from build123d import *
from OCP.BRepFilletAPI import BRepFilletAPI_MakeFillet
from build123d.topology import SkipClean

# Parameters (mm, degrees)
SKETCH2_R               = 43
SKETCH2_R_2             = 40
BOSS_EXTRUDE1_DEPTH     = 48
SKETCH3_R               = 40
BOSS_EXTRUDE2_DEPTH     = 8.5
CUT_EXTRUDE1_DEPTH      = 71.924255371
CUT_EXTRUDE1_DEPTH_BACK = 71.924255371
SKETCH4_W               = 41
SKETCH4_H               = 21
CUT_EXTRUDE2_DEPTH      = 5
BOSS_EXTRUDE3_START     = 3
SKETCH6_W               = 120
SKETCH6_H               = 110
SKETCH6_R               = 40
BOSS_EXTRUDE3_DEPTH     = 3
FILLET1_R               = 3
FILLET1_R_2             = 1
SKETCH7_R               = 2.1
SKETCH7_W               = 8
SKETCH7_H               = 4
CUT_EXTRUDE3_DEPTH      = 3


with BuildPart() as part:
    # Sketch2 → Boss-Extrude1 (new body)
    with BuildSketch(Plane(origin=(0, 0, 0), x_dir=(1, 0, 0), z_dir=(0, 1, 0))):
        with Locations(Location((0, 0, 0), (0, 0, 270))):
            Circle(SKETCH2_R)
        with Locations(Location((0, 0, 0), (0, 0, 270))):
            Circle(SKETCH2_R_2, mode=Mode.SUBTRACT)
    extrude(amount=BOSS_EXTRUDE1_DEPTH)

    # Sketch3 → Boss-Extrude2 (add)
    with BuildSketch(Plane(origin=(0, 28, 0), x_dir=(1, 0, 0), z_dir=(0, 1, 0))):
        with Locations(Location((0, 0, 0), (0, 0, 270))):
            Circle(SKETCH3_R)
    extrude(amount=BOSS_EXTRUDE2_DEPTH)

    # Sketch4 → Cut-Extrude1 (cut, two sides: drawn at the far end of the back side and taken through both)
    with BuildSketch(Plane(origin=(0, 36.5, 0), x_dir=(1, 0, 0), z_dir=(0, 1, 0)).offset(-CUT_EXTRUDE1_DEPTH_BACK)):
        with BuildLine():
            Line((14, 6.75), (16, 6.75))
            ThreePointArc((16, 6.75), (17.75, 5), (16, 3.25))
            Line((16, 3.25), (14, 3.25))
            ThreePointArc((14, 3.25), (12.25, 5), (14, 6.75))
        make_face()
        with Locations((-10, 0)):
            Rectangle(SKETCH4_W, SKETCH4_H)
        with BuildLine():
            Line((-36, 6.75), (-34, 6.75))
            ThreePointArc((-34, 6.75), (-32.25, 5), (-34, 3.25))
            Line((-34, 3.25), (-36, 3.25))
            ThreePointArc((-36, 3.25), (-37.75, 5), (-36, 6.75))
        make_face()
        with BuildLine():
            Line((-36, -3.25), (-34, -3.25))
            ThreePointArc((-34, -3.25), (-32.25, -5), (-34, -6.75))
            Line((-34, -6.75), (-36, -6.75))
            ThreePointArc((-36, -6.75), (-37.75, -5), (-36, -3.25))
        make_face()
        with BuildLine():
            Line((14, -6.75), (16, -6.75))
            ThreePointArc((16, -6.75), (17.75, -5), (16, -3.25))
            Line((16, -3.25), (14, -3.25))
            ThreePointArc((14, -3.25), (12.25, -5), (14, -6.75))
        make_face()
    extrude(amount=CUT_EXTRUDE1_DEPTH + CUT_EXTRUDE1_DEPTH_BACK, mode=Mode.SUBTRACT)

    # Sketch5 → Cut-Extrude2 (cut)
    with BuildSketch(Plane(origin=(43, 0, 0), x_dir=(0, 0, -1), z_dir=(1, 0, 0))):
        with BuildLine():
            Line((-6, 17), (6, 17))
            ThreePointArc((6, 17), (8, 15), (6, 13))
            Line((6, 13), (-6, 13))
            ThreePointArc((-6, 13), (-8, 15), (-6, 17))
        make_face()
    extrude(amount=-CUT_EXTRUDE2_DEPTH, mode=Mode.SUBTRACT)

    # Sketch6 → Boss-Extrude3 (add)
    with SkipClean():  # the faces are left unmerged after this step: merging them gives an invalid solid
        with BuildSketch(Plane.XZ.offset(BOSS_EXTRUDE3_START)):
            Rectangle(SKETCH6_W, SKETCH6_H)
            with Locations(Location((0, 0, 0), (0, 0, 270))):
                Circle(SKETCH6_R, mode=Mode.SUBTRACT)
        extrude(amount=-BOSS_EXTRUDE3_DEPTH)

    # Fillet1
    fillet1_edges_1 = [part.edges().sort_by_distance(p)[0] for p in [
        (0, 48, -43),
        (0, 0, -43),
    ]]
    fillet1_edges_2 = [part.edges().sort_by_distance(p)[0] for p in [
        (0, 0, 55),
        (60, 0, 0),
        (-60, 0, 0),
        (0, 0, -55),
    ]]
    fillet1 = BRepFilletAPI_MakeFillet(part.part.solid().wrapped)
    for e in fillet1_edges_1:
        fillet1.Add(FILLET1_R - 0.0001, e.wrapped)
    for e in fillet1_edges_2:
        fillet1.Add(FILLET1_R_2 - 0.0001, e.wrapped)
    add(Compound.cast(fillet1.Shape()), mode=Mode.REPLACE)  # a hair under: the kernel refuses the full size

    # Sketch7 → Cut-Extrude3 (cut)
    with BuildSketch(Plane(origin=(0, 0, 0), x_dir=(1, 0, 0), z_dir=(0, 1, 0))):
        with Locations(Location((-41.5, 43, 0), (0, 0, 270))):
            Circle(SKETCH7_R)
        with Locations(Location((43.5, 22.5, 0), (0, 0, 270))):
            Circle(SKETCH7_R)
        with Locations(Location((43.5, -22.5, 0), (0, 0, 270))):
            Circle(SKETCH7_R)
        with Locations(Location((-41.5, -43, 0), (0, 0, 270))):
            Circle(SKETCH7_R)
        with Locations(Location((48.1, 0, 0), (0, 0, 270))):
            Circle(SKETCH7_R)
        with Locations((-49, 25.6)):
            Rectangle(SKETCH7_W, SKETCH7_H)
        with Locations((-49, 18)):
            Rectangle(SKETCH7_W, SKETCH7_H)
        with Locations((-49, 33.2)):
            Rectangle(SKETCH7_W, SKETCH7_H)
        with Locations((-49, 40.8)):
            Rectangle(SKETCH7_W, SKETCH7_H)
        with Locations((-49, -40.8)):
            Rectangle(SKETCH7_W, SKETCH7_H)
        with Locations((-49, -33.2)):
            Rectangle(SKETCH7_W, SKETCH7_H)
        with Locations((-49, -25.6)):
            Rectangle(SKETCH7_W, SKETCH7_H)
        with Locations((-49, -18)):
            Rectangle(SKETCH7_W, SKETCH7_H)
    extrude(amount=-CUT_EXTRUDE3_DEPTH, mode=Mode.SUBTRACT)


solid = part.part
Input: part model. Units: mm. Frame: model coordinates. A direction names the side the tool comes from. Round coordinates to 2 decimals unless told otherwise and drop trailing zeros. Loops run counter-clockwise (first coordinate to the right, second up) from the corner with the lowest first, then second, coordinate; pieces in that order, holes last. Notation, with made-up numbers: M 35,-12 L 51,-12 A8 ccw 51,-4 Z; hole C 42,48.25 d11. An arc over 180 degrees is marked long. Answer as CSV lines item,"result". Start each with the question number.
(1) Line query: line 1 (X direction, y = -1.25, z = 0); line 2 (X direction, y = 19.25, z = 0); line 3 (Y direction, x = -36, z = 46.5). Output: solid intervals per line, ascending. Write a range as [from, to].
(2) Section C-C, the plane y = 6. Output: boundary loops of the cut face in (x, z), plus the area to 3 significant figures.
(3) Draft query along Z for faces 4 (the flat face through (-53, -1, 26)), 5 (the flat face through (-40, 0, 25)), 6 (the flat face through (-49, -1, -38.8)). Return one class per face: released by +Z, released by -Z, zero draft, split by the parting line, or undercut.
(4) First-contact query: pin 1 (2 mm diameter, centred on x = 3, y = 13, fed in from -Z); pin 2 (5 mm diameter, centred on x = -46, y = 3, fed in from +Z); pin 3 (3 mm diameter, centred on x = 0, y = 29, fed in from -Z); pin 4 (8 mm diameter, centred on y = 24.5, z = -8.5, fed in from -X). Flat tips, straight axial feed; report the tip coordinate or a pass-through.
(5) Section D-D, the plane x = -41.5. State how many separate pieces and enclosed holes the cut face has, plus the area to 3 significant figures.
(6) Section A-A, the plane x = 48.1. Output: boundary loops of the cut face in (y, z).
(7) Section B-B, the plane y = 34.5. Output: boundary loops of the cut face in (x, z).
(8) Reachability of faces 1 (the cylindrical face through (41, 15, 8)), 2 (the flat face through (1, 36.5, 17)), 3 (the flat face through (-45, -1, -41)) from +Z, -Z, +X, -X, +Y, -Y: full face, straight path, thin tool, end or side. Return the list, or none.
Values found:
1,line 1,"x = [-60, -40], [40, 46], [50.2, 60]"
1,line 2,"x = [-43, -40], [40, 43]"
1,line 3,"y = [-3, 0]"
2,outline,"C 0,0 d86; hole C 0,0 d80"
2,area,"782 mm²"
3,face 4,"undercut"
3,face 5,"zero draft"
3,face 6,"undercut"
4,pin 1,"stops at z = -42.95"
4,pin 2,"passes through"
4,pin 3,"stops at z = -43"
4,pin 4,"stops at x = -42.76"
5,separate pieces,"3"
5,enclosed holes,"0"
5,area,"1,380 mm²"
6,outline,"M -3,-55 L -1,-55 A1 ccw 0,-54 L 0,-2.1 L -3,-2.1 Z; M -3,2.1 L 0,2.1 L 0,54 A1 ccw -1,55 L -3,55 Z"
7,outline,"C 0,0 d86; hole M -36,-6.75 L -34,-6.75 A1.75 ccw -34,-3.25 L -36,-3.25 A1.75 ccw Z; hole M -36,3.25 L -34,3.25 A1.75 ccw -34,6.75 L -36,6.75 A1.75 ccw Z; hole M -30.5,-10.5 L 10.5,-10.5 L 10.5,10.5 L -30.5,10.5 Z; hole M 14,-6.75 L 16,-6.75 A1.75 ccw 16,-3.25 L 14,-3.25 A1.75 ccw Z; hole M 14,3.25 L 16,3.25 A1.75 ccw 16,6.75 L 14,6.75 A1.75 ccw Z"
8,face 1,"+X"
8,face 2,"+Y"
8,face 3,"+Y, -Y"
